Check sheet for the modelled part. Datum: model origin and axes. Units: mm. Face numbers are marked on the shaded views. A direction names the side the tool comes from. Give positions to 0.01 mm unless a question says otherwise; leave off trailing zeros. Order: outer loops, then holes, each group sorted by start corner. A loop starts at its lowest first (then second) coordinate and runs counter-clockwise, first axis right, second up.
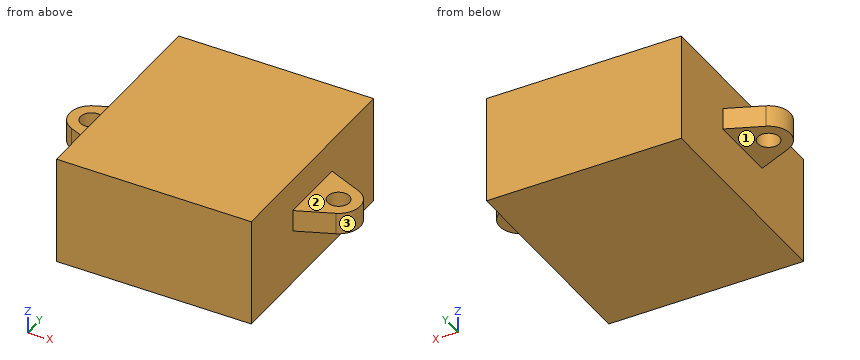
```python
from build123d import *

# Parameters (mm, degrees)
SKETCH1_W           = 27
SKETCH1_H           = 30
BOSS_EXTRUDE3_DEPTH = 15
SKETCH5_R           = 1.5
BOSS_EXTRUDE7_DEPTH = 3


with BuildPart() as part:
    # Sketch1 → Boss-Extrude3 (new body)
    with BuildSketch(Plane.XY):
        with Locations((-43.997662922, -20.897486093)):
            Rectangle(SKETCH1_W, SKETCH1_H)
    extrude(amount=BOSS_EXTRUDE3_DEPTH)

    # Sketch5 → Boss-Extrude7 (add)
    with BuildSketch(Plane.XY.offset(7.5)):
        with BuildLine():
            Line((-30.497662922, -16.097486093), (-25.697662922, -18.13623415))
            ThreePointArc((-25.697662922, -18.13623415), (-23.870474804, -20.897486093), (-25.697662922, -23.658738035))
            Line((-25.697662922, -23.658738035), (-30.497662922, -25.697486093))
            Line((-30.497662922, -25.697486093), (-30.497662922, -16.097486093))
        make_face()
        with Locations((-26.870474804, -20.897486093)):
            Circle(SKETCH5_R, mode=Mode.SUBTRACT)
        with BuildLine():
            Line((-57.497662922, -16.097486093), (-57.497662922, -25.697486093))
            Line((-57.497662922, -25.697486093), (-62.297662922, -23.658738035))
            ThreePointArc((-62.297662922, -23.658738035), (-64.12485104, -20.897486093), (-62.297662922, -18.13623415))
            Line((-62.297662922, -18.13623415), (-57.497662922, -16.097486093))
        make_face()
        with Locations((-61.12485104, -20.897486093)):
            Circle(SKETCH5_R, mode=Mode.SUBTRACT)
    extrude(amount=BOSS_EXTRUDE7_DEPTH)


solid = part.part
```
(1) Cross-section at B-B on z = 8.25. Enter the section's corners in (x, y), then the cut area to 3 significant figures.
Response values:
outline: (-62.3, -23.66) - (-57.5, -25.7) - (-57.5, -35.9) - (-30.5, -35.9) - (-30.5, -25.7) - (-25.7, -23.66) arc R3 ccw to (-25.7, -18.14) - (-30.5, -16.1) - (-30.5, -5.9) - (-57.5, -5.9) - (-57.5, -16.1) - (-62.3, -18.14) arc R3 ccw to start; hole circle Ø3 at (-61.12, -20.9); hole circle Ø3 at (-26.87, -20.9)
area: 883 mm2
(2) Cross-section at D-D on z = 2. Enter the section's corners in (x, y).
Response values:
outline: (-57.5, -35.9) - (-30.5, -35.9) - (-30.5, -5.9) - (-57.5, -5.9) - close
(3) Material ranges on L1, parallel to X at y = -19.25, z = 1.75; L2, parallel to Z at x = -29.5, y = -22.5; L3, parallel to Y at x = -26, z = 9.25, recorded low to high.
Response values:
L1: x = -57.5 to -30.5
L2: z = 7.5 to 10.5
L3: y = -23.79 to -22.12, -19.68 to -18.01
(4) Gauge pin test, flat ends, axial feed: pin 1 Ø5.5 at (x, y) = (-27.5, -19) entering from -Z; pin 2 Ø7.5 at (y, z) = (-28, 4.5) entering from +X; pin 3 Ø7.5 at (x, y) = (-61, -20) entering from +Z; pin 4 Ø4.5 at (y, z) = (-25, 5) entering from -X. Record the tip position at first contact, or that the pin passes through.
Response values:
pin 1: stops at z = 7.5
pin 2: stops at x = -30.5
pin 3: stops at z = 15
pin 4: stops at x = -57.5
(5) Set-up check for the marked faces 1, 2 and 3: record each of +Z, -Z, +X, -X, +Y, -Y from which the full face is reachable in a straight line by a thin tool's end or side.
Response values:
face 1: -Z, -X, +Y, -Y
face 2: +Z, +X, +Y, -Y
face 3: +Z, -Z, +X
(6) Cross-section at C-C on y = -33.5. Enter the section's corners in (x, z).
Response values:
outline: (-57.5, 0) - (-30.5, 0) - (-30.5, 15) - (-57.5, 15) - close
(7) Cross-section at A-A on x = -27.5. Enter the section's corners in (y, z).
Response values:
outline: (-24.42, 7.5) - (-22.26, 7.5) - (-22.26, 10.5) - (-24.42, 10.5) - close; (-19.54, 7.5) - (-17.37, 7.5) - (-17.37, 10.5) - (-19.54, 10.5) - close
